Check sheet for the modelled part. Datum: model origin and axes. Units: mm. A direction names the side the tool comes from. Give positions to 0.01 mm unless a question says otherwise; leave off trailing zeros. Loops run counter-clockwise (first coordinate to the right, second up) from the corner with the lowest first, then second, coordinate; pieces in that order, holes last. Notation, with made-up numbers: (20, 43) -> (35, 43) arc R34 ccw to (35, 82) -> close; hole circle Ø9 at (14.5, -27.75). An arc over 180 degrees is marked (long way). Write each question's results on one line, items separated by ' | '. Start each with the question number.
Item 1: Scan lines: line 1 along Y through (x, z) = (230.5, 3); line 2 along X through (y, z) = (6.5, 2.5); line 3 along Z through (x, y) = (131, -0.5). Record each from-to range of solid material in increasing order.
Item 2: Cross-section at B-B on z = 8.25. Enter the section's corners in (x, y), then the cut area to 3 significant figures.
Item 3: Mould release check, pull along Y, two halves, no side actions. Record for faces 6 (the face through (114, 6, 0)), 7 (the face through (214.88, 0.07, -8.54)), 8 (the face through (132.52, 8.54, -0.07)): pulls with the +Y half, pulls with the -Y half, needs draft (parallel to the pull), parting line crosses it, or undercut.
Item 4: Cross-section at A-A on y = 0. Enter the section's corners in (x, z).
Item 5: Cross-section at C-C on x = 83.5. Enter the section's corners in (y, z).
Item 6: Access from +Z, -Z, +X, -X, +Y, -Y to the whole of each face (thin tool, end or side, straight path). Record for faces 1 (the face through (124.413, -3.304, 10.492)), 2 (the face through (196, 0, -6)), 3 (the face through (114, -8, 3)), 4 (the face through (114, 8, -3)), 5 (the face through (196, -3, 8)).
Item 7: Gauge pin test, flat ends, axial feed: pin 1 Ø2.5 at (x, y) = (115, -8.5) entering from +Z; pin 2 Ø5 at (x, y) = (109, 8.5) entering from +Z; pin 3 Ø3 at (x, y) = (102.5, -1) entering from +Z; pin 4 Ø3 at (x, z) = (121.5, -4) entering from +Y. Record the tip position at first contact, or that the pin passes through.
from build123d import *

# Parameters (mm, degrees)
SKETCH1_W           = 140
SKETCH1_H           = 11
CUT_EXTRUDE1_DEPTH  = 5
SKETCH5_R           = 11
BOSS_EXTRUDE1_DEPTH = 97.36
CUT_EXTRUDE2_DEPTH  = 5
SKETCH8_R           = 11
BOSS_EXTRUDE2_DEPTH = 15


with BuildPart() as part:
    # Sketch1 → Revolve1 (revolve)
    with BuildSketch(Plane.XY, mode=Mode.PRIVATE) as revolve1_sk:
        with Locations((70, 5.5)):
            Rectangle(SKETCH1_W, SKETCH1_H)
    revolve(revolve1_sk.sketch.rotate(Axis((0, 0, 0), (1, 0, 0)), 90), axis=Axis((0, 0, 0), (1, 0, 0)))

    # Sketch4 → Cut-Extrude1 (cut)
    with BuildSketch(Plane(origin=(0, 11, 0), x_dir=(1, 0, 0), z_dir=(0, 1, 0))):
        with BuildLine():
            Line((129.52, -3), (98.12, -3))
            ThreePointArc((98.12, -3), (95.12, 0), (98.12, 3))
            Line((98.12, 3), (129.52, 3))
            ThreePointArc((129.52, 3), (132.52, 0), (129.52, -3))
        make_face()
    cut_extrude1 = extrude(amount=-CUT_EXTRUDE1_DEPTH, mode=Mode.SUBTRACT)

    # Mirror1: Cut-Extrude1 across plane
    add(cut_extrude1.mirror(Plane.ZX), mode=Mode.SUBTRACT)

    # Sketch5 → Boss-Extrude1 (add)
    with BuildSketch(Plane(origin=(140, 0, 0), x_dir=(0, 0, -1), z_dir=(1, 0, 0))):
        with Locations(Location((0, 0, 0), (0, 0, 180))):
            Circle(SKETCH5_R)
    extrude(amount=BOSS_EXTRUDE1_DEPTH)

    # Sketch7 → Cut-Extrude2 (cut)
    with BuildSketch(Plane.XY.offset(11)):
        with BuildLine():
            Line((211.88, -3), (180.48, -3))
            ThreePointArc((180.48, -3), (177.48, 0), (180.48, 3))
            Line((180.48, 3), (211.88, 3))
            ThreePointArc((211.88, 3), (214.88, 0), (211.88, -3))
        make_face()
    cut_extrude2 = extrude(amount=-CUT_EXTRUDE2_DEPTH, mode=Mode.SUBTRACT)

    # Mirror2: Cut-Extrude2 across plane
    add(cut_extrude2.mirror(Plane.XY), mode=Mode.SUBTRACT)

    # Sketch8 → Boss-Extrude2 (add)
    with BuildSketch(Plane(origin=(237.36, 0, 0), x_dir=(0, 0, -1), z_dir=(1, 0, 0))):
        with Locations(Location((0, 0, 0), (0, 0, 180))):
            Circle(SKETCH8_R)
    extrude(amount=BOSS_EXTRUDE2_DEPTH)


solid = part.part
Answer sheet:
1) line 1: y = -10.58 to 10.58 | line 2: x = 0 to 96.46, 131.18 to 252.36 | line 3: z = -10.99 to 10.99
2) outline: (0, -7.28) -> (252.36, -7.28) -> (252.36, 7.28) -> (0, 7.28) -> close; hole (180.48, -3) -> (211.88, -3) arc R3 ccw to (211.88, 3) -> (180.48, 3) arc R3 ccw to start | area: 3,460 mm²
3) face 6: pulls with the +Y half | face 7: undercut | face 8: needs draft
4) outline: (0, -11) -> (177.48, -11) -> (177.48, -6) -> (214.88, -6) -> (214.88, -11) -> (252.36, -11) -> (252.36, 11) -> (214.88, 11) -> (214.88, 6) -> (177.48, 6) -> (177.48, 11) -> (0, 11) -> close
5) outline: circle Ø22 at (0, 0)
6) face 1: +X, -X | face 2: -Z | face 3: -Y | face 4: +Y | face 5: +Z
7) pin 1: stops at z = 8.27 | pin 2: stops at z = 9.22 | pin 3: stops at z = 11 | pin 4: stops at y = 10.58
